The model under review builds one solid part; all positions refer to its coordinate system, in mm. A direction names the side the tool comes from. Give positions to 0.01 mm unless a question says otherwise; leave off trailing zeros. Write each loop counter-clockwise with the first axis right and the second up, starting at its lowest first coordinate (ties: lowest second). Pieces come first, ordered by that corner, then holes. Notation, with made-up numbers: M -39,-29 L -19,-29 A28 ccw -19,9 Z; hole C 6.25,7.25 d7. An arc over 180 degrees is marked long. Write each question's results on one line, items separated by ' | '. Start each with the question number.
from build123d import *

# Parameters (mm, degrees)
ESBO_O4_R                = 6.1
ESBO_O4_R_2              = 4.75
RESSALTO_EXTRUS_O3_DEPTH = 9.2
ESBO_O4_3_R              = 8
ESBO_O4_3_R_2            = 6.1
RESSALTO_EXTRUS_O4_DEPTH = 1
RESSALTO_EXTRUS_O6_START = -1
ESBO_O5_R                = 8
ESBO_O5_R_2              = 4.75
RESSALTO_EXTRUS_O6_DEPTH = 1
FILETE5_R                = 0.2
FILETE6_R                = 0.2


with BuildPart() as part:
    # Esbo_o4 → Ressalto-extrus_o3 (new body)
    with BuildSketch(Plane(origin=(0, 0, 0), x_dir=(1, 0, 0), z_dir=(0, 1, 0))):
        with Locations(Location((0, 0, 0), (0, 0, 270))):
            Circle(ESBO_O4_R)
        with Locations(Location((0, 0, 0), (0, 0, 270))):
            Circle(ESBO_O4_R_2, mode=Mode.SUBTRACT)
    extrude(amount=RESSALTO_EXTRUS_O3_DEPTH)

    # Esbo_o4_3 → Ressalto-extrus_o4 (add)
    with BuildSketch(Plane(origin=(0, 0, 0), x_dir=(1, 0, 0), z_dir=(0, 1, 0))):
        with Locations(Location((0, 0, 0), (0, 0, 270))):
            Circle(ESBO_O4_3_R)
        with Locations(Location((0, 0, 0), (0, 0, 270))):
            Circle(ESBO_O4_3_R_2, mode=Mode.SUBTRACT)
    extrude(amount=RESSALTO_EXTRUS_O4_DEPTH)

    # Esbo_o5 → Ressalto-extrus_o6 (add)
    with BuildSketch(Plane(origin=(0, 9.2, 0), x_dir=(1, 0, 0), z_dir=(0, 1, 0)).offset(RESSALTO_EXTRUS_O6_START)):
        with Locations(Location((0, 0, 0), (0, 0, 270))):
            Circle(ESBO_O5_R)
        with Locations(Location((0, 0, 0), (0, 0, 270))):
            Circle(ESBO_O5_R_2, mode=Mode.SUBTRACT)
    extrude(amount=RESSALTO_EXTRUS_O6_DEPTH)

    # Filete5
    filete5_edges = [part.edges().sort_by_distance(p)[0] for p in [
        (0, 8.2, -8),
        (0, 9.2, -8),
    ]]
    fillet(filete5_edges, radius=FILETE5_R)

    # Filete6
    filete6_edges = [part.edges().sort_by_distance(p)[0] for p in [
        (0, 0, -8),
        (0, 1, -8),
    ]]
    fillet(filete6_edges, radius=FILETE6_R)


solid = part.part
(1) Add section A-A (z = 0). State the section outline as (x, y) points, then the cut area to 3 significant figures.
(2) Machinability: for faces 4 (the flat face through (-4, 8.2, -5)), 5 (the flat face through (-3, 0, -4)), which of the approach directions +Z, -Z, +X, -X, +Y, -Y give a long, thin tool a straight path to every point of the face, cutting with its end or side? Answer none if there is none.
(3) Add section C-C (y = 8.75). State the section outline as (x, z) points, then the cut area to 3 significant figures.
(4) Clearance check with flat-ended pins moving along their axes: P1, Ø2, axis at x = 6, y = 1.5, coming from the -Z side; P2, Ø5, axis at x = 6.5, y = 1.5, coming from the +Z side; P3, Ø3, axis at x = -1.5, y = 7, coming from the +Z side. State where each tip first meets the part, or that it passes through.
(5) Wall thickness on L1, parallel to Y at x = 6.75, z = 1.5; L2, parallel to X at y = 7, z = 0; L3, parallel to Z at x = -0.25, y = 8: over which ranges is each line inside the solid? List them lowest first.
(6) Draft analysis for pull direction Z (two halves, no side actions). For faces 1 (the flat face through (-4, 1, -5)), 2 (the cylindrical face through (-7.81, 0.5, -1.73)), 3 (the cylindrical face through (-2.89, 4.54, -3.77)), state which applies: pulls with the +Z half, pulls with the -Z half, needs draft (parallel to the pull), parting line crosses it, or undercut.
(7) Add section B-B (x = 0). State the section outline as (y, z) points.
(8) Add section D-D (y = 7.5). State the section outline as (x, z) points, then the cut area to 3 significant figures.
Calculated:
1) outline: M -8,0.2 A0.2 ccw -7.8,0 L -4.75,0 L -4.75,9.2 L -7.8,9.2 A0.2 ccw -8,9 L -8,8.4 A0.2 ccw -7.8,8.2 L -6.1,8.2 L -6.1,1 L -7.8,1 A0.2 ccw -8,0.8 Z; M 4.75,0 L 7.8,0 A0.2 ccw 8,0.2 L 8,0.8 A0.2 ccw 7.8,1 L 6.1,1 L 6.1,8.2 L 7.8,8.2 A0.2 ccw 8,8.4 L 8,9 A0.2 ccw 7.8,9.2 L 4.75,9.2 Z | area: 32.4 mm²
2) face 4: none | face 5: +Z, -Z, +X, -X, -Y
3) outline: C 0,0 d16; hole C 0,0 d9.5 | area: 130 mm²
4) P1: stops at z = -6.04 | P2: stops at z = 6.87 | P3: stops at z = 7.95
5) L1: y = 0 to 1, 8.2 to 9.2 | L2: x = -6.1 to -4.75, 4.75 to 6.1 | L3: z = -6.09 to -4.74, 4.74 to 6.09
6) face 1: needs draft | face 2: parting line crosses it | face 3: undercut
7) outline: M 0,-7.8 A0.2 ccw 0.2,-8 L 0.8,-8 A0.2 ccw 1,-7.8 L 1,-6.1 L 8.2,-6.1 L 8.2,-7.8 A0.2 ccw 8.4,-8 L 9,-8 A0.2 ccw 9.2,-7.8 L 9.2,-4.75 L 0,-4.75 Z; M 0,4.75 L 9.2,4.75 L 9.2,7.8 A0.2 ccw 9,8 L 8.4,8 A0.2 ccw 8.2,7.8 L 8.2,6.1 L 1,6.1 L 1,7.8 A0.2 ccw 0.8,8 L 0.2,8 A0.2 ccw 0,7.8 Z
8) outline: C 0,0 d12.2; hole C 0,0 d9.5 | area: 46.0 mm²
